from build123d import *

# Parameters (mm, degrees)
BOSS_EXTRU_2_DEPTH      = 18
ENL_V_MAT_EXTRU_1_DEPTH = 19
CONG_1_R                = 7


with BuildPart() as part:
    # Esquisse2 → Boss.-Extru.2 (new body)
    with BuildSketch(Plane.XY):
        with BuildLine():
            Line((0, 0), (100, 0))
            Line((100, 0), (100, 45.254412261))
            ThreePointArc((100, 45.254412261), (99.813462099, 46.607402512), (99.267766953, 47.859439178))
            ThreePointArc((99.267766953, 47.859439178), (100, 54), (106.140560822, 54.732233047))
            ThreePointArc((106.140560822, 54.732233047), (107.392597488, 54.186537901), (108.745587739, 54))
            Line((108.745587739, 54), (130, 54))
            Line((130, 54), (130, 360))
            Line((130, 360), (-30.494949366, 360))
            Line((-30.494949366, 360), (-30.494949366, 101.23368794))
            ThreePointArc((-30.494949366, 101.23368794), (-32.612333247, 92.044193475), (-38.537502558, 84.707812102))
            ThreePointArc((-38.537502558, 84.707812102), (-39.242879856, 83.834433367), (-39.494949366, 82.740445931))
            Line((-39.494949366, 82.740445931), (-39.494949366, 54))
            Line((-39.494949366, 54), (-8.745587739, 54))
            ThreePointArc((-8.745587739, 54), (-7.392597488, 54.186537901), (-6.140560822, 54.732233047))
            ThreePointArc((-6.140560822, 54.732233047), (0, 54), (0.732233047, 47.859439178))
            ThreePointArc((0.732233047, 47.859439178), (0.186537901, 46.607402512), (0, 45.254412261))
            Line((0, 45.254412261), (0, 0))
        make_face()
    extrude(amount=BOSS_EXTRU_2_DEPTH)

    # Esquisse1 → Enlèv. mat.-Extru.1 (cut, through all)
    with BuildSketch(Plane.XY):
        with BuildLine():
            Line((59.5, 28.248771852), (59.5, 25.751228148))
            ThreePointArc((59.5, 25.751228148), (59.599672829, 25.160561143), (59.88765279, 24.635309084))
            ThreePointArc((59.88765279, 24.635309084), (59.5, 18), (52.864690916, 17.61234721))
            ThreePointArc((52.864690916, 17.61234721), (52.339438857, 17.900327171), (51.748771852, 18))
            Line((51.748771852, 18), (48.251228148, 18))
            ThreePointArc((48.251228148, 18), (47.660561143, 17.900327171), (47.135309084, 17.61234721))
            ThreePointArc((47.135309084, 17.61234721), (40.5, 18), (40.11234721, 24.635309084))
            ThreePointArc((40.11234721, 24.635309084), (40.400327171, 25.160561143), (40.5, 25.751228148))
            Line((40.5, 25.751228148), (40.5, 28.248771852))
            ThreePointArc((40.5, 28.248771852), (40.400327171, 28.839438857), (40.11234721, 29.364690916))
            ThreePointArc((40.11234721, 29.364690916), (40.5, 36), (47.135309084, 36.38765279))
            ThreePointArc((47.135309084, 36.38765279), (47.660561143, 36.099672829), (48.251228148, 36))
            Line((48.251228148, 36), (51.748771852, 36))
            ThreePointArc((51.748771852, 36), (52.339438857, 36.099672829), (52.864690916, 36.38765279))
            ThreePointArc((52.864690916, 36.38765279), (59.5, 36), (59.88765279, 29.364690916))
            ThreePointArc((59.88765279, 29.364690916), (59.599672829, 28.839438857), (59.5, 28.248771852))
        make_face()
    extrude(amount=ENL_V_MAT_EXTRU_1_DEPTH, mode=Mode.SUBTRACT)

    # Congé1
    cong_1_edges = [part.edges().sort_by_distance(p)[0] for p in [
        (-39.494949366, 54, 9),
        (130, 54, 9),
        (100, 0, 9),
        (0, 0, 9),
    ]]
    fillet(cong_1_edges, radius=CONG_1_R)

    # Symétrie1: part across plane


with BuildPart() as part_1:
    add(part.part)
    add(part.part.mirror(Plane(origin=(130, 360, 18), x_dir=(0, 0, 1), z_dir=(0, -1, 0))))


solid = part_1.part
Work out the finished part from the listing and answer in its coordinate system (mm). A direction names the side the tool comes from. Coordinates: 2 decimals unless noted, no trailing zeros. Loops run counter-clockwise (first coordinate to the right, second up) from the corner with the lowest first, then second, coordinate; pieces in that order, holes last. Notation, with made-up numbers: M 25,-10.75 L 55,-10.75 A19 ccw 55,-1.75 Z; hole C -23,81.5 d2. An arc over 180 degrees is marked long. Answer in a Markdown table with one row per item. Add a question column.
1. Find section B-B, the plane y = 456. Write down the section's boundary in (x, z).
2. The mould has two halves that part along Y. Classify faces 4 (the flat face through (-30.495, 356, 9)), 5 (the flat face through (-21, 54, 9)), 6 (the flat face through (130, 364, 9)): pulls with the +Y half, pulls with the -Y half, needs draft (parallel to the pull), parting line crosses it, or undercut.
3. Flat-ended cylindrical pins translate along their axes: P1, Ø5.5, axis at x = -26, z = 13, coming from the +Y side; P2, Ø5.5, axis at y = 694, z = 5, coming from the +X side; P3, Ø1, axis at y = 98.5, z = 14.5, coming from the -X side. Find the tip coordinate at first contact, or state that the pin passes through.
4. Consider L1, parallel to Y at x = 54, z = 11.25; L2, parallel to X at y = 247, z = 2.25; L3, parallel to Y at x = 58, z = 3.75. Determine where each line is inside the solid, lowest interval first.
5. Find section C-C, the plane z = 5.5. State how many separate pieces and enclosed holes the cut face has, then the cut area to 3 significant figures.
6. A tool of negligible diameter and unlimited length cuts with its end or side. For faces 1 (the flat face through (116, 666, 9)), 2 (the flat face through (0, 694, 9)), 3 (the flat face through (116, 54, 9)), from which of +Z, -Z, +X, -X, +Y, -Y can it reach the whole face along a straight path? Write none if from no direction.
7. Find section A-A, the plane x = -23. Write down the section's boundary in (y, z), then the cut area to 3 significant figures.
Reported:
| question | item | result |
|---|---|---|
| 1 | outline | M -30.49,0 L 130,0 L 130,18 L -30.49,18 Z |
| 2 | face 4 | undercut |
| 2 | face 5 | pulls with the -Y half |
| 2 | face 6 | needs draft |
| 3 | P1 | stops at y = 666 |
| 3 | P2 | stops at x = 100 |
| 3 | P3 | stops at x = -30.75 |
| 4 | L1 | y = 0 to 16.94, 37.06 to 682.94, 703.06 to 720 |
| 4 | L2 | x = -30.49 to 130 |
| 4 | L3 | y = 0 to 16.97, 37.03 to 682.97, 703.03 to 720 |
| 5 | separate pieces | 1 |
| 5 | enclosed holes | 2 |
| 5 | area | 109,000 mm^2 |
| 6 | face 1 | +Z, -Z, +X, +Y |
| 6 | face 2 | +Z, -Z, -X, +Y |
| 6 | face 3 | +Z, -Z, +X, -Y |
| 7 | outline | M 54,0 L 666,0 L 666,18 L 54,18 Z |
| 7 | area | 11,000 mm^2 |
